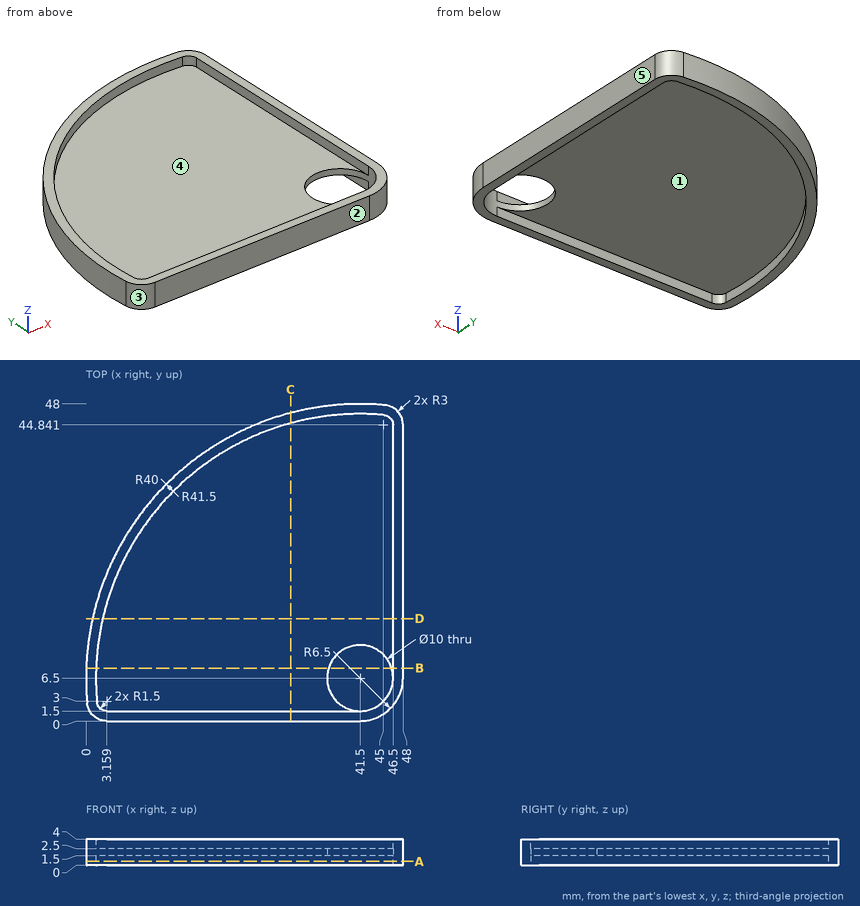
The figure shows three views and two pictorial views of one solid part (mm, origin at its lowest corner). Answer the questions. A direction names the side the tool comes from. Round coordinates to 2 decimals unless told otherwise and drop trailing zeros. Loops run counter-clockwise (first coordinate to the right, second up) from the corner with the lowest first, then second, coordinate; pieces in that order, holes last. Notation, with made-up numbers: (-32.75, -32) - (4.25, -32) arc R20 ccw to (4.25, -27) - close; hole circle Ø9 at (-15.5, 62.5). An arc over 180 degrees is marked (long way). Use one line per item in the form item = value. Start each with the question number.
(1) Find section D-D on y = 15.5. Determine the outline of the cut face in (x, z) (1 decimal).
(2) Consider line 1 (Y direction, x = 41.5, z = 2.65); line 2 (Y direction, x = 41.5, z = 2). Determine where each line is inside the solid, lowest interval first.
(3) Which of the six approach directions +Z, -Z, +X, -X, +Y, -Y give full straight-line access (tool end or side, diameter ignored) to the marked faces 4 and 5?
(4) Determine the mould class of the marked faces 1, 2 and 3 for opening direction X: +X half, -X half, draft (parallel to the pull), parting line (faces both ways), or undercut.
(5) Find section A-A on z = 0.6. Determine the outline of the cut face in (x, y) (1 decimal).
(6) Flat-ended cylindrical pins translate along their axes: P1, Ø0.8, axis at y = 19.5, z = 1, coming from the -X side; P2, Ø0.8, axis at x = 30, z = 3.5, coming from the +Y side; P3, Ø1.6, axis at x = 15, z = 0.5, coming from the +Y side (1 decimal); P4, Ø10, axis at x = 14.5, y = 30.5, coming from the -Z side. Find the tip coordinate at first contact, or state that the pin passes through.
(7) Find section C-C on x = 31. Determine the outline of the cut face in (y, z).
(8) Find section B-B on y = 8. Determine the outline of the cut face in (x, z).
Answer list:
q1.outline = (1, 0) - (2.5, 0) - (2.5, 1.5) - (46.5, 1.5) - (46.5, 0) - (48, 0) - (48, 4) - (46.5, 4) - (46.5, 2.5) - (2.5, 2.5) - (2.5, 4) - (1, 4) - close
q2.line_1 = 0 to 1.5, 46.5 to 48
q2.line_2 = 0 to 1.5, 11.5 to 48
q3.face_4 = +Z
q3.face_5 = +Z, -Z, +X, +Y, -Y
q4.face_1 = undercut
q4.face_2 = draft
q4.face_3 = -X half
q5.outline = (0.2, 2.7) arc R3 ccw to (3.2, 0) - (41.5, 0) arc R6.5 ccw to (48, 6.5) - (48, 44.8) arc R3 ccw to (45.3, 47.8) arc R41.5 ccw to start; hole (1.7, 2.9) arc R1.5 ccw to (3.2, 1.5) - (41.5, 1.5) arc R5 ccw to (46.5, 6.5) - (46.5, 44.8) arc R1.5 ccw to (45.1, 46.3) arc R40 ccw to start
q6.P1 = 1.96
q6.P2 = 46.49
q6.P3 = 39.1
q6.P4 = 0
q7.outline = (0, 0) - (1.5, 0) - (1.5, 1.5) - (45.1, 1.5) - (45.1, 0) - (46.65, 0) - (46.65, 4) - (45.1, 4) - (45.1, 2.5) - (1.5, 2.5) - (1.5, 4) - (0, 4) - close
q8.outline = (0.03, 0) - (1.53, 0) - (1.53, 1.5) - (36.73, 1.5) - (36.73, 2.5) - (1.53, 2.5) - (1.53, 4) - (0.03, 4) - close; (46.27, 1.5) - (46.5, 1.5) - (46.5, 0) - (48, 0) - (48, 4) - (46.5, 4) - (46.5, 2.5) - (46.27, 2.5) - close
